```python
from build123d import *

# Parameters (mm, degrees)
BOSS_EXTRUDE1_DEPTH = 4
SKETCH3_R           = 17.5
CUT_EXTRUDE1_DEPTH  = 2
CUT_EXTRUDE2_DEPTH  = 2


with BuildPart() as part:
    # Sketch1 → Boss-Extrude1 (new body)
    with BuildSketch(Plane(origin=(0, 0, 0), x_dir=(1, 0, 0), z_dir=(0, 1, 0))):
        with BuildLine():
            Line((2.5, -72.247448714), (-2.5, -72.247448714))
            Line((-2.5, -72.247448714), (-2.5, -12.247448714))
            ThreePointArc((-2.5, -12.247448714), (0, 12.5), (2.5, -12.247448714))
            Line((2.5, -12.247448714), (2.5, -72.247448714))
        make_face()
    extrude(amount=BOSS_EXTRUDE1_DEPTH)

    # Sketch3 → Cut-Extrude1 (cut)
    with BuildSketch(Plane(origin=(0, 4, 0), x_dir=(1, 0, 0), z_dir=(0, 1, 0))):
        Circle(SKETCH3_R)
    extrude(amount=-CUT_EXTRUDE1_DEPTH, mode=Mode.SUBTRACT)

    # Sketch4 → Cut-Extrude2 (cut)
    with BuildSketch(Plane(origin=(0, 4, 0), x_dir=(1, 0, 0), z_dir=(0, 1, 0))):
        with BuildLine():
            Line((-0.65, -17.487924405), (-0.65, -72.247448714))
            Line((-0.65, -72.247448714), (0.65, -72.247448714))
            Line((0.65, -72.247448714), (0.65, -17.487924405))
            ThreePointArc((0.65, -17.487924405), (0, -17.5), (-0.65, -17.487924405))
        make_face()
    extrude(amount=-CUT_EXTRUDE2_DEPTH, mode=Mode.SUBTRACT)


solid = part.part
```
Here's how the part is built. I have some questions about the finished solid (model axes, mm). A direction names the side the tool comes from. Round coordinates to 2 decimals unless told otherwise and drop trailing zeros. Order: outer loops, then holes, each group sorted by start corner. A loop starts at its lowest first (then second) coordinate and runs counter-clockwise, first axis right, second up. Notation, with made-up numbers: M 82.25,59.25 L 88.25,59.25 A24 cw 88.25,79.25 Z; hole C -7.5,50.25 d10. An arc over 180 degrees is marked long. Use CSV: the item, a comma, the result in double quotes.
1) I want a section at C-C (x = 10.5). List the corners of the cut face in (y, z) for me.
Taken from the geometry:
outline,"M 0,-6.78 L 2,-6.78 L 2,6.78 L 0,6.78 Z"
2) I want a section at D-D (z = 0). List the corners of the cut face in (x, y) for me, then the cut area to 3 significant figures.
Taken from the geometry:
outline,"M -12.5,0 L 12.5,0 L 12.5,2 L -12.5,2 Z"
area,"50.0 mm^2"
3) If we mould it in two halves opening along X, with no side actions, what happens to faces 6 (the cylindrical face through (-0.51, 0.99, -12.49)), 7 (the flat face through (2, 4, 44)), 8 (the cylindrical face through (1.56, 3.01, 17.43))? For each: pulls with the +X half, pulls with the -X half, needs draft (parallel to the pull), parting line crosses it, or undercut.
Taken from the geometry:
face 6,"parting line crosses it"
face 7,"needs draft"
face 8,"undercut"
4) I'm going to push flat-ended pins straight in: P1, Ø1.6, axis at y = 3, z = 42, coming from the +X side; P2, Ø2, axis at x = -4, y = 2.5, coming from the -Z side; P3, Ø1, axis at y = 3.5, z = 51, coming from the -X side. Where does each tip first touch, or does it pass through?
Taken from the geometry:
P1,"x = 2.5"
P2,"z = -12.1"
P3,"x = -2.5"
5) I want a section at B-B (z = 63.5). List the corners of the cut face in (x, y) for me, then the cut area to 3 significant figures.
Taken from the geometry:
outline,"M -2.5,0 L 2.5,0 L 2.5,4 L 0.65,4 L 0.65,2 L -0.65,2 L -0.65,4 L -2.5,4 Z"
area,"17.4 mm^2"
6) I want a section at A-A (y = 3.2). List the corners of the cut face in (x, z) for me, then the cut area to 3 significant figures.
Taken from the geometry:
outline,"M -2.5,17.32 A17.5 cw -0.65,17.49 L -0.65,72.25 L -2.5,72.25 Z; M 0.65,17.49 A17.5 cw 2.5,17.32 L 2.5,72.25 L 0.65,72.25 Z"
area,"203 mm^2"
7) On a 3-axis mill with a long thin cutter (end or side, diameter ignored), from which of +Z, -Z, +X, -X, +Y, -Y can I reach the whole of each face in a straight line? I mean faces 1 (the cylindrical face through (-1.59, 3.014, 17.428)), 2 (the flat face through (-2.5, 2, 43)), 3 (the flat face through (0, 0, 17)), 4 (the flat face through (2.5, 2, 42)), 5 (the flat face through (0.65, 3, 45)). Say none if no direction works.
Taken from the geometry:
face 1,"-Z, +Y"
face 2,"+Z, -X, +Y, -Y"
face 3,"+Z, -Z, +X, -X, -Y"
face 4,"+Z, +X, +Y, -Y"
face 5,"+Z, -Z, +Y"
8) I need wall thicknesses on line 1 along X through (y, z) = (2.3, 38); line 2 along Z through (x, y) = (-1, 3.7). Which ranges of each line are inside material? Lowest first, please. Write a range as [from, to].
Taken from the geometry:
line 1,"[-2.5, -0.65], [0.65, 2.5]"
line 2,"[17.47, 72.25]"
